Geometry: final body of the model. Coordinates: model frame, mm. Give positions to 0.01 mm unless a question says otherwise; leave off trailing zeros. Loops run counter-clockwise (first coordinate to the right, second up) from the corner with the lowest first, then second, coordinate; pieces in that order, holes last.
from build123d import *

# Parameters (mm, degrees)
F0_R     = 12.7
F1_DEPTH = 19.05


with BuildPart() as f1:
    # F0 (on Front) → F1 (new body)
    with BuildSketch(Plane.XZ):
        with BuildLine():
            Line((12.5552676618, 50.8), (6.35, 50.8))
            ThreePointArc((6.35, 50.8), (0, 44.45), (-6.35, 50.8))
            Line((-6.35, 50.8), (-12.7, 50.8))
            ThreePointArc((-12.7, 50.8), (-12.6547477412, 50.1030744688), (-12.623195922, 49.4053944235))
            ThreePointArc((-12.623195922, 49.4053944235), (-0.5027005097, 38.1099530262), (12.4733220574, 48.4112269151))
            ThreePointArc((12.4733220574, 48.4112269151), (12.4943375608, 49.6062980822), (12.5552676618, 50.8))
        make_face()
        with BuildLine():
            ThreePointArc((-6.35, 50.8), (0, 57.15), (6.35, 50.8))
            Line((6.35, 50.8), (12.5552676618, 50.8))
            Line((12.5552676618, 50.8), (12.7, 50.8))
            ThreePointArc((12.7, 50.8), (0, 63.5), (-12.7, 50.8))
            Line((-12.7, 50.8), (-6.35, 50.8))
        make_face()
        with BuildLine():
            Line((12.7, 50.8), (12.5552676618, 50.8))
            ThreePointArc((12.5552676618, 50.8), (12.4943375608, 49.6062980822), (12.4733220574, 48.4112269151))
            ThreePointArc((12.4733220574, 48.4112269151), (12.6432035127, 49.6002479693), (12.7, 50.8))
        make_face()
        with BuildLine():
            ThreePointArc((-12.623195922, 49.4053944235), (-12.6547477412, 50.1030744688), (-12.7, 50.8))
            ThreePointArc((-12.7, 50.8), (-12.6807844436, 50.1016405688), (-12.623195922, 49.4053944235))
        make_face()
        with BuildLine():
            ThreePointArc((49.4621205903, 12.6293340555), (23.373403019, 22.6698095536), (12.4733220574, 48.4112269151))
            ThreePointArc((12.4733220574, 48.4112269151), (-0.5027005097, 38.1099530262), (-12.623195922, 49.4053944235))
            ThreePointArc((-12.623195922, 49.4053944235), (-23.0125550108, 23.0125550108), (-49.4053944235, 12.623195922))
            ThreePointArc((-49.4053944235, 12.623195922), (-41.3395166397, 8.4728539813), (-38.1, 0))
            ThreePointArc((-38.1, 0), (-41.2035577614, -8.3185513379), (-48.9973695056, -12.571416917))
            ThreePointArc((-48.9973695056, -12.571416917), (-22.7523388598, -22.7523388598), (-12.571416917, -48.9973695056))
            ThreePointArc((-12.571416917, -48.9973695056), (0.2857229322, -38.1032144853), (12.6397809271, -49.5647113232))
            ThreePointArc((12.6397809271, -49.5647113232), (23.1125114369, -23.1125114369), (49.5647113232, -12.6397809271))
            ThreePointArc((49.5647113232, -12.6397809271), (38.1001046657, -0.0515606332), (49.4621205903, 12.6293340555))
        make_face()
        Circle(F0_R, mode=Mode.SUBTRACT)
        with BuildLine():
            ThreePointArc((50.8, 12.7), (50.1313911561, 12.6584030193), (49.4621205903, 12.6293340555))
            ThreePointArc((49.4621205903, 12.6293340555), (38.1001046657, -0.0515606332), (49.5647113232, -12.6397809271))
            ThreePointArc((49.5647113232, -12.6397809271), (50.1826156034, -12.6645582134), (50.8, -12.7))
            Line((50.8, -12.7), (50.8, -6.35))
            ThreePointArc((50.8, -6.35), (44.45, 0), (50.8, 6.35))
            Line((50.8, 6.35), (50.8, 12.7))
        make_face()
        with BuildLine():
            ThreePointArc((50.8, 12.7), (50.1301278125, 12.6823212092), (49.4621205903, 12.6293340555))
            ThreePointArc((49.4621205903, 12.6293340555), (50.1313911561, 12.6584030193), (50.8, 12.7))
        make_face()
        with BuildLine():
            ThreePointArc((-50.8, 12.7), (-50.1030744688, 12.6547477412), (-49.4053944235, 12.623195922))
            ThreePointArc((-49.4053944235, 12.623195922), (-50.1016405688, 12.6807844436), (-50.8, 12.7))
        make_face()
        with BuildLine():
            ThreePointArc((-38.1, 0), (-41.3395166397, 8.4728539813), (-49.4053944235, 12.623195922))
            ThreePointArc((-49.4053944235, 12.623195922), (-50.1030744688, 12.6547477412), (-50.8, 12.7))
            Line((-50.8, 12.7), (-50.8, 6.35))
            ThreePointArc((-50.8, 6.35), (-46.3098719395, 4.4901280605), (-44.45, 0))
            ThreePointArc((-44.45, 0), (-46.3098719395, -4.4901280605), (-50.8, -6.35))
            Line((-50.8, -6.35), (-50.8, -12.7))
            ThreePointArc((-50.8, -12.7), (-49.8995176161, -12.6240323908), (-48.9973695056, -12.571416917))
            ThreePointArc((-48.9973695056, -12.571416917), (-41.2035577614, -8.3185513379), (-38.1, 0))
        make_face()
        with BuildLine():
            ThreePointArc((63.5, 0), (59.7802561211, 8.9802561211), (50.8, 12.7))
            Line((50.8, 12.7), (50.8, 6.35))
            ThreePointArc((50.8, 6.35), (55.2901280605, 4.4901280605), (57.15, 0))
            ThreePointArc((57.15, 0), (55.2901280605, -4.4901280605), (50.8, -6.35))
            Line((50.8, -6.35), (50.8, -12.7))
            ThreePointArc((50.8, -12.7), (59.7802561211, -8.9802561211), (63.5, 0))
        make_face()
        with BuildLine():
            ThreePointArc((50.8, -12.7), (50.1826156034, -12.6645582134), (49.5647113232, -12.6397809271))
            ThreePointArc((49.5647113232, -12.6397809271), (50.1816221924, -12.6849362981), (50.8, -12.7))
        make_face()
        with BuildLine():
            Line((-50.8, 6.35), (-50.8, 12.7))
            ThreePointArc((-50.8, 12.7), (-63.5, 0), (-50.8, -12.7))
            Line((-50.8, -12.7), (-50.8, -6.35))
            ThreePointArc((-50.8, -6.35), (-57.15, 0), (-50.8, 6.35))
        make_face()
        with BuildLine():
            ThreePointArc((12.7, -50.8), (12.6645582134, -50.1826156034), (12.6397809271, -49.5647113232))
            ThreePointArc((12.6397809271, -49.5647113232), (0.2857229322, -38.1032144853), (-12.571416917, -48.9973695056))
            ThreePointArc((-12.571416917, -48.9973695056), (-12.6240323908, -49.8995176161), (-12.7, -50.8))
            Line((-12.7, -50.8), (-6.35, -50.8))
            ThreePointArc((-6.35, -50.8), (0, -44.45), (6.35, -50.8))
            Line((6.35, -50.8), (12.7, -50.8))
        make_face()
        with BuildLine():
            ThreePointArc((12.7, -50.8), (12.6849362981, -50.1816221924), (12.6397809271, -49.5647113232))
            ThreePointArc((12.6397809271, -49.5647113232), (12.6645582134, -50.1826156034), (12.7, -50.8))
        make_face()
        with BuildLine():
            ThreePointArc((-50.8, -12.7), (-49.8963946784, -12.6678134429), (-48.9973695056, -12.571416917))
            ThreePointArc((-48.9973695056, -12.571416917), (-49.8995176161, -12.6240323908), (-50.8, -12.7))
        make_face()
        with BuildLine():
            ThreePointArc((-12.7, -50.8), (0, -63.5), (12.7, -50.8))
            Line((12.7, -50.8), (6.35, -50.8))
            ThreePointArc((6.35, -50.8), (0, -57.15), (-6.35, -50.8))
            Line((-6.35, -50.8), (-12.7, -50.8))
        make_face()
        with BuildLine():
            ThreePointArc((-12.7, -50.8), (-12.6240323908, -49.8995176161), (-12.571416917, -48.9973695056))
            ThreePointArc((-12.571416917, -48.9973695056), (-12.6678134429, -49.8963946784), (-12.7, -50.8))
        make_face()
    extrude(amount=F1_DEPTH)


solid = f1.part
Item 1: Section query C-C on y = -17.5. Return loops of the section in (x, z).
Values follow:
outline: (-49.41, 12.62) arc R12.7 ccw (long way) to (-49, -12.57) arc R34.88 cw to (-12.57, -49) arc R12.7 ccw (long way) to (12.64, -49.56) arc R35.82 cw to (49.56, -12.64) arc R12.7 ccw (long way) to (49.46, 12.63) arc R35.77 cw to (12.47, 48.41) arc R12.7 ccw (long way) to (-12.62, 49.41) arc R35.55 cw to start; hole circle Ø12.7 at (-50.8, 0); hole circle Ø25.4 at (0, 0); hole circle Ø12.7 at (0, -50.8); hole circle Ø12.7 at (0, 50.8); hole circle Ø12.7 at (50.8, 0)
Item 2: Pin query (flat end, axial travel): pin 1 (2 mm diameter, centred on x = -33, y = -5, fed in from -Z); pin 2 (1.5 mm diameter, centred on x = -7.5, y = -10.5, fed in from -Z); pin 3 (23 mm diameter, centred on x = 0, z = 0, fed in from -Y); pin 4 (8 mm diameter, centred on x = -47, y = -13, fed in from -Z). Return the tip coordinate at first contact, or that it passes through.
Values follow:
pin 1: stops at z = -16.13
pin 2: stops at z = -61.56
pin 3: passes through
pin 4: stops at z = -12.82
Item 3: Ray query, probe 1 along Z at (x, y) = (0, -6); probe 2 along Z at (x, y) = (51, -16); probe 3 along Z at (x, y) = (-11.5, -10). Return the intervals inside material, ascending.
Values follow:
probe 1: z = -63.5 to -57.15, -44.45 to -12.7, 12.7 to 44.45, 57.15 to 63.5
probe 2: z = -12.7 to -6.35, 6.35 to 12.7
probe 3: z = -56.19 to -5.39, 5.39 to 56.19
Item 4: Draft query along Z for faces 1 (the face through (0, 0, 14)), 2 (the face through (-2.75, -9.39, -12.4)). Return one class per face: +Z half, -Z half, draft (parallel to the pull), parting line (faces both ways), or undercut.
Values follow:
face 1: draft
face 2: undercut
Item 5: Section query B-B on z = -2. Return loops of the section in (x, y), plus the area to 3 significant figures.
Values follow:
outline: (-63.34, -19.05) - (-56.83, -19.05) - (-56.83, 0) - (-63.34, 0) - close; (-44.77, -19.05) - (-12.54, -19.05) - (-12.54, 0) - (-44.77, 0) - close; (12.54, -19.05) - (44.77, -19.05) - (44.77, 0) - (12.54, 0) - close; (56.83, -19.05) - (63.34, -19.05) - (63.34, 0) - (56.83, 0) - close
area: 1,480 mm2
Item 6: Section query D-D on x = -27. Return loops of the section in (y, z).
Values follow:
outline: (-19.05, -19.14) - (0, -19.14) - (0, 19.58) - (-19.05, 19.58) - close
Item 7: Section query A-A on x = 0. Return loops of the section in (y, z).
Values follow:
outline: (-19.05, -63.5) - (0, -63.5) - (0, -57.15) - (-19.05, -57.15) - close; (-19.05, -44.45) - (0, -44.45) - (0, -12.7) - (-19.05, -12.7) - close; (-19.05, 12.7) - (0, 12.7) - (0, 44.45) - (-19.05, 44.45) - close; (-19.05, 57.15) - (0, 57.15) - (0, 63.5) - (-19.05, 63.5) - close
